Autodesk Inventor part; units mm, degrees
ref_plane "Work Plane1" through (0, 0, 1.25) normal (0, 0, 1) x (1, 0, 0)
ref_plane "YZ Plane" through (0, 0, 0) normal (1, 0, 0) x (0, 1, 0)
ref_plane "XZ Plane" through (0, 0, 0) normal (0, 1, 0) x (-1, 0, 0)
sketch "Sketch1" plane through (0, 0, 0) normal (0, 0, 1) x (1, 0, 0)
  circle A0 centre (0, 0) radius 5
  dimension "d0" = 10
extrude "Extrusion1" add sketch "Sketch1" along normal blind 2.5
hole "Hole1" at (0, 0, 2.5) direction (0, 0, -1) diameter 6 end through all
sketch "Sketch2" plane through (0, 0, 2.5) normal (0, 0, 1) x (1, 0, 0)
  circle A0 centre (0, 0) radius 4.5
  circle A1 centre (0, 0) radius 3.5
  dimension "d12" = 9
  dimension "d13" = 7
extrude "Extrusion2" cut sketch "Sketch2" against normal blind 0.5
ref_plane "Work Plane1" through (0, 0, 1.25) normal (0, 0, 1) x (1, 0, 0)
mirror "Mirror1" about plane through (0, 0, 1.25) normal (0, 0, 1) of "Extrusion2"
properties part number "bearing_6x10x2,5" material "Stainless Steel"
For this review, take the finished solid that the model builds, in its own axes (mm). A direction names the side the tool comes from. Round coordinates to 2 decimals unless told otherwise and drop trailing zeros. Write each loop counter-clockwise with the first axis right and the second up, starting at its lowest first coordinate (ties: lowest second). Pieces come first, ordered by that corner, then holes. Notation, with made-up numbers: M -8.75,-3.75 L 29.25,-3.75 A23 ccw 29.25,21.25 Z; hole C -8.5,22.5 d9. An arc over 180 degrees is marked long. One line per item, written item: value. Start each with the question number.
(1) Machinability: for faces 1 (the cylindrical face through (-0.59, 4.46, 2.25)), 2 (the flat face through (3, 1, 2.5)), 3 (the flat face through (0, -4, 0.5)), which of the approach directions +Z, -Z, +X, -X, +Y, -Y give a long, thin tool a straight path to every point of the face, cutting with its end or side? Answer none if there is none.
(2) The part is to be moulded in two halves that separate along X. For faces 4 (the flat face through (0, -4, 2)), 5 (the flat face through (3, 1, 0)), 6 (the cylindrical face through (-1.08, 4.88, 1.23)), say which applies: released by +X, released by -X, zero draft, split by the parting line, or undercut.
(3) We need section A-A (x = 0). Give the boundary of the cut face in (y, z), and give its area (3 significant figures).
(4) Wall thickness on line 1 (Y direction, x = 0, z = 0.35); line 2 (Y direction, x = 0, z = 0.85); line 3 (Y direction, x = -1.5, z = 0.15): over which ranges is each line inside the solid? List them lowest first.
(5) Insertion check: pin 1 (3 mm diameter, centred on x = -3, y = 2, fed in from +Z); pin 2 (1.5 mm diameter, centred on x = 1.5, z = 0.5, fed in from -Y); pin 3 (1.5 mm diameter, centred on y = 2, z = 1.5, fed in from +X). Each pin has a flat end and moves straight along its axis. Give the tip position at first contact, or say it passes through.
(6) We need section D-D (y = 3.25). Give the boundary of the cut face in (x, z), and give its area (3 significant figures).
(7) We need section C-C (z = 0.2). Give the boundary of the cut face in (x, y).
Result:
1. face 1: +Z
1. face 2: +Z, +X, -X, +Y, -Y
1. face 3: -Z
2. face 4: undercut
2. face 5: zero draft
2. face 6: split by the parting line
3. outline: M -5,0 L -4.5,0 L -4.5,0.5 L -3.5,0.5 L -3.5,0 L -3,0 L -3,2.5 L -3.5,2.5 L -3.5,2 L -4.5,2 L -4.5,2.5 L -5,2.5 Z; M 3,0 L 3.5,0 L 3.5,0.5 L 4.5,0.5 L 4.5,0 L 5,0 L 5,2.5 L 4.5,2.5 L 4.5,2 L 3.5,2 L 3.5,2.5 L 3,2.5 Z
3. area: 8.00 mm²
4. line 1: -5 to -4.5, -3.5 to -3, 3 to 3.5, 4.5 to 5
4. line 2: -5 to -3, 3 to 5
4. line 3: -4.77 to -4.24, -3.16 to -2.6, 2.6 to 3.16, 4.24 to 4.77
5. pin 1: z = 2.5
5. pin 2: y = -4.94
5. pin 3: x = 4.84
6. outline: M -3.8,0 L -3.11,0 L -3.11,0.5 L -1.3,0.5 L -1.3,0 L 1.3,0 L 1.3,0.5 L 3.11,0.5 L 3.11,0 L 3.8,0 L 3.8,2.5 L 3.11,2.5 L 3.11,2 L 1.3,2 L 1.3,2.5 L -1.3,2.5 L -1.3,2 L -3.11,2 L -3.11,2.5 L -3.8,2.5 Z
6. area: 15.4 mm²
7. outline: C 0,0 d10; C 0,0 d7; hole C 0,0 d9; hole C 0,0 d6
